```python
from build123d import *

# Parameters (mm, degrees)
SKETCH_1_W               = 30
SKETCH_1_H               = 30
EXTRUDE_1_DEPTH          = 2
SKETCH_2_W               = 10.2
SKETCH_2_H               = 2
CUT_EXTRUDE_1_DEPTH      = 2.5
CUT_EXTRUDE_3_DEPTH      = 43
CHAMFER_1_SIZE           = 1.5
CUT_EXTRUDE_4_DEPTH      = 0.5
FILLET_1_R               = 1
CUT_EXTRUDE_2_DEPTH      = 43
CUT_EXTRUDE_2_DEPTH_BACK = 43
SKETCH_3_R               = 0.65
CUT_EXTRUDE_7_DEPTH      = 0.5
CUT_EXTRUDE_8_DEPTH      = 10
CUT_EXTRUDE_9_DEPTH      = 10
CHAMFER_2_SIZE           = 1
CUT_EXTRUDE_10_DEPTH     = 10


with BuildPart() as part:
    # 草图1 → 凸台-拉伸1 (new body)
    with BuildSketch(Plane.XY):
        Rectangle(SKETCH_1_W, SKETCH_1_H)
    extrude(amount=EXTRUDE_1_DEPTH)

    # 草图2 → 切除-拉伸1 (cut)
    with BuildSketch(Plane(origin=(0, 15, 0), x_dir=(1, 0, 0), z_dir=(0, 1, 0))):
        with Locations((0, -1)):
            Rectangle(SKETCH_2_W, SKETCH_2_H)
    extrude(amount=-CUT_EXTRUDE_1_DEPTH, mode=Mode.SUBTRACT)

    # 草图4 → 切除-拉伸3 (cut)
    with BuildSketch(Plane(origin=(0, 0, 0), x_dir=(-1, 0, 0), z_dir=(0, 0, -1))):
        Polygon((-10, -13.5), (-8.5, -15), (-10, -15), (-15, -15), (-15, -13.5), align=None)
    extrude(amount=-CUT_EXTRUDE_3_DEPTH, mode=Mode.SUBTRACT)

    # 倒角1
    chamfer_1_edges = [part.edges().sort_by_distance(p)[0] for p in [
        (15, -13.5, 1),
    ]]
    chamfer(chamfer_1_edges, length=CHAMFER_1_SIZE)

    # 草图5 → 切除-拉伸4 (cut)
    with BuildSketch(Plane(origin=(0, 0, 0), x_dir=(-1, 0, 0), z_dir=(0, 0, -1))):
        Polygon((-15, -12), (-5, -12), (-2, -15), (-8.5, -15), (-10, -13.5), (-13.5, -13.5), align=None)
    extrude(amount=-CUT_EXTRUDE_4_DEPTH, mode=Mode.SUBTRACT)

    # 圆角1
    fillet_1_edges = [part.edges().sort_by_distance(p)[0] for p in [
        (10.05, 15, 2),
        (10.05, 15, 0),
        (-10.05, 15, 2),
        (-10.05, 15, 0),
        (0, 12.5, 2),
        (0, 12.5, 0),
    ]]
    fillet(fillet_1_edges, radius=FILLET_1_R - 0.0001)  # a hair under: the kernel refuses the full size

    # 草图3 → 切除-拉伸2 (cut, two sides: drawn at the far end of the back side and taken through both)
    with BuildSketch(Plane(origin=(-5.1, 0, 0), x_dir=(0, 0, -1), z_dir=(1, 0, 0)).offset(-CUT_EXTRUDE_2_DEPTH_BACK)):
        with Locations(Location((-1, 14, 0), (0, 0, 180))):
            Circle(SKETCH_3_R)
    extrude(amount=CUT_EXTRUDE_2_DEPTH + CUT_EXTRUDE_2_DEPTH_BACK, mode=Mode.SUBTRACT)

    # 草图9 → 切除-拉伸7 (cut)
    with BuildSketch(Plane(origin=(0, 0, 0), x_dir=(-1, 0, 0), z_dir=(0, 0, -1))):
        with BuildLine():
            Line((-2.293324317, -12.585355339), (-0.407968978, -14.470710678))
            ThreePointArc((-0.407968978, -14.470710678), (-0.375526643, -14.492387953), (-0.3372583, -14.5))
            Line((-0.3372583, -14.5), (1.500609665, -14.5))
            ThreePointArc((1.500609665, -14.5), (1.546803642, -14.469134172), (1.535965005, -14.414644661))
            Line((1.535965005, -14.414644661), (-0.349390335, -12.529289322))
            ThreePointArc((-0.349390335, -12.529289322), (-0.381832669, -12.507612047), (-0.420101013, -12.5))
            Line((-0.420101013, -12.5), (-2.257968978, -12.5))
            ThreePointArc((-2.257968978, -12.5), (-2.304162955, -12.530865828), (-2.293324317, -12.585355339))
        make_face()
        with BuildLine():
            Line((2.579898987, -12.5), (0.742031022, -12.5))
            ThreePointArc((0.742031022, -12.5), (0.695837045, -12.530865828), (0.706675683, -12.585355339))
            Line((0.706675683, -12.585355339), (2.592031022, -14.470710678))
            ThreePointArc((2.592031022, -14.470710678), (2.624473357, -14.492387953), (2.6627417, -14.5))
            Line((2.6627417, -14.5), (4.500609665, -14.5))
            ThreePointArc((4.500609665, -14.5), (4.546803642, -14.469134172), (4.535965005, -14.414644661))
            Line((4.535965005, -14.414644661), (2.650609665, -12.529289322))
            ThreePointArc((2.650609665, -12.529289322), (2.618167331, -12.507612047), (2.579898987, -12.5))
        make_face()
        with BuildLine():
            Line((5.579898987, -12.5), (3.742031022, -12.5))
            ThreePointArc((3.742031022, -12.5), (3.695837045, -12.530865828), (3.706675683, -12.585355339))
            Line((3.706675683, -12.585355339), (5.592031022, -14.470710678))
            ThreePointArc((5.592031022, -14.470710678), (5.624473357, -14.492387953), (5.6627417, -14.5))
            Line((5.6627417, -14.5), (7.500609665, -14.5))
            ThreePointArc((7.500609665, -14.5), (7.546803642, -14.469134172), (7.535965005, -14.414644661))
            Line((7.535965005, -14.414644661), (5.650609665, -12.529289322))
            ThreePointArc((5.650609665, -12.529289322), (5.618167331, -12.507612047), (5.579898987, -12.5))
        make_face()
    extrude(amount=-CUT_EXTRUDE_7_DEPTH, mode=Mode.SUBTRACT)

    # 草图10 → 切除-拉伸8 (cut)
    with BuildSketch(Plane(origin=(0, 0, 0), x_dir=(-1, 0, 0), z_dir=(0, 0, -1))):
        with BuildLine():
            Line((8.026955262, -12.95), (11.6, -12.95))
            ThreePointArc((11.6, -12.95), (11.882842712, -13.067157288), (12, -13.35))
            Line((12, -13.35), (12, -14.05))
            ThreePointArc((12, -14.05), (11.882842712, -14.332842712), (11.6, -14.45))
            Line((11.6, -14.45), (8.726955262, -14.45))
            ThreePointArc((8.726955262, -14.45), (8.573881889, -14.419551813), (8.44411255, -14.332842712))
            Line((8.44411255, -14.332842712), (7.74411255, -13.632842712))
            ThreePointArc((7.74411255, -13.632842712), (7.657403449, -13.196926627), (8.026955262, -12.95))
        make_face()
    extrude(amount=-CUT_EXTRUDE_8_DEPTH, mode=Mode.SUBTRACT)

    # 草图11 → 切除-拉伸9 (cut)
    with BuildSketch(Plane(origin=(0, 0, 0), x_dir=(-1, 0, 0), z_dir=(0, 0, -1))):
        Polygon((15, -7), (13.5, -8.5), (13.5, -15), (15, -15), align=None)
    extrude(amount=-CUT_EXTRUDE_9_DEPTH, mode=Mode.SUBTRACT)

    # 倒角2
    chamfer_2_edges = [part.edges().sort_by_distance(p)[0] for p in [
        (-13.5, -15, 1),
    ]]
    chamfer(chamfer_2_edges, length=CHAMFER_2_SIZE)

    # 草图12 → 切除-拉伸10 (cut)
    with BuildSketch(Plane(origin=(0, 0, 0), x_dir=(-1, 0, 0), z_dir=(0, 0, -1))):
        Polygon((10, 15), (10, 13), (13, 10), (15, 8), (15, 15), align=None)
    cut_extrude_10 = extrude(amount=-CUT_EXTRUDE_10_DEPTH, mode=Mode.SUBTRACT)

    # 镜向4: 切除-拉伸10 across plane
    add(cut_extrude_10.mirror(Plane(origin=(0, 0, 0), x_dir=(0, 0, 1), z_dir=(1, 0, 0))), mode=Mode.SUBTRACT)


solid = part.part
```
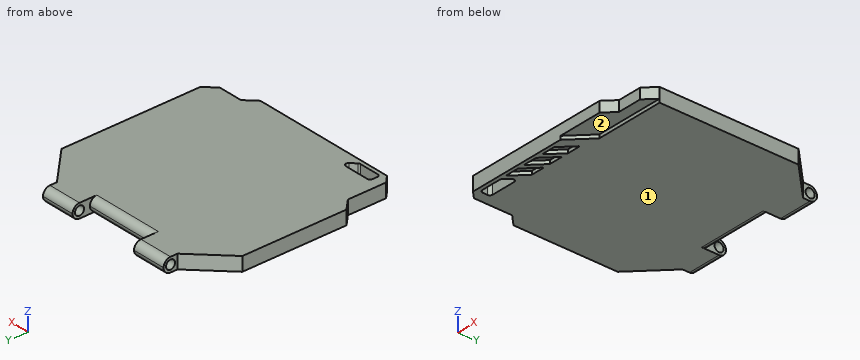
Design review of the part built by this model. Coordinates are the model's own, in mm. Face numbers are marked on the shaded views. A direction names the side the tool comes from. Coordinates: 2 decimals unless noted, no trailing zeros. Order: outer loops, then holes, each group sorted by start corner. A loop starts at its lowest first (then second) coordinate and runs counter-clockwise, first axis right, second up. Notation, with made-up numbers: M 50,-25.75 L 73,-25.75 A14 ccw 73,-16.75 Z; hole C -26,35.5 d2. An arc over 180 degrees is marked long. Answer as a JSON object with one key per item and string values. Group by question number.
1) Tool access review of the marked faces 1 and 2: name each direction out of +Z, -Z, +X, -X, +Y, -Y from which nothing blocks a thin tool from reaching the whole face with its end or side.
2) For pin 1 (1.2 mm diameter, centred on y = 14, z = 1, fed in from +X); pin 2 (0.9 mm diameter, centred on x = 10, y = -13.5, fed in from -Z); pin 3 (1 mm diameter, centred on y = -11.5, z = 1, fed in from -X); pin 4 (1.2 mm diameter, centred on x = 12, z = 1, fed in from -Y), all flat-tipped, find the tip position at first contact; note any pin that passes through.
3) Add section C-C, the plane x = 13. Write out the cut boundary in (y, z), then the cut area to 4 significant figures.
4) Add section A-A, the plane x = -9.25. Count the separate pieces of the cut face and the enclosed holes in it, then the cut area to 3 significant figures.
5) Wall thickness on L1, parallel to Y at x = -8.7, z = 1; L2, parallel to Y at x = -6.95, z = 1; L3, parallel to X at y = -13.5, z = 0.1: over which ranges is each line inside the solid? List them lowest first.
Computed values:
{
 "1": {"face 1": "-Z, +X, -X, +Y, -Y", "face 2": "-Z, +X, -Y"},
 "2": {"pin 1": "passes through", "pin 2": "stops at z = 0.5", "pin 3": "stops at x = -13.5", "pin 4": "stops at y = -13.5"},
 "3": {"outline": "M -13.5,0.5 L -12,0.5 L -12,0 L 10,0 L 10,2 L -13.5,2 Z", "area": "46.25 mm^2"},
 "4": {"separate pieces": "2", "enclosed holes": "1", "area": "55.2 mm^2"},
 "5": {"L1": "y = -15 to -14.45, -12.95 to 13.35, 14.65 to 15", "L2": "y = -15 to 13.35, 14.65 to 15", "L3": "x = -13.5 to -12, -7.66 to -6.62, -4.62 to -3.62, -1.62 to -0.62, 1.38 to 3.5"}
}
